```python
from build123d import *

# Parameters (mm, degrees)
BOSS_EXTRUDE1_DEPTH = 127
SKETCH4_W           = 31.75
SKETCH4_H           = 76.2
CUT_EXTRUDE3_DEPTH  = 63.5
SKETCH5_W           = 31.75
SKETCH5_H           = 76.2
CUT_EXTRUDE4_DEPTH  = 63.246
CUT_EXTRUDE6_DEPTH  = 69.85
CUT_EXTRUDE8_DEPTH  = 69.85
SKETCH9_R           = 4.7625
CUT_EXTRUDE9_DEPTH  = 461.057390442


with BuildPart() as part:
    # Sketch1 → Boss-Extrude1 (new body)
    with BuildSketch(Plane.XY):
        Polygon((63.5, -381), (63.5, 381), (31.75, 381), (31.75, 431.8), (-31.75, 431.8), (-31.75, 381), (-63.5, 381), (-63.5, -381), align=None)
    extrude(amount=-BOSS_EXTRUDE1_DEPTH)

    # Sketch4 → Cut-Extrude3 (cut)
    with BuildSketch(Plane.ZY.offset(63.5)):
        with Locations((-47.625, -215.9)):
            Rectangle(SKETCH4_W, SKETCH4_H)
    extrude(amount=-CUT_EXTRUDE3_DEPTH, mode=Mode.SUBTRACT)

    # Sketch5 → Cut-Extrude4 (cut)
    with BuildSketch(Plane(origin=(0, 0, -127), x_dir=(-1, 0, 0), z_dir=(0, 0, -1))):
        with Locations((-15.875, -215.9)):
            Rectangle(SKETCH5_W, SKETCH5_H)
    extrude(amount=-CUT_EXTRUDE4_DEPTH, mode=Mode.SUBTRACT)

    # Sketch7 → Cut-Extrude6 (cut)
    with BuildSketch(Plane(origin=(63.5, 0, 0), x_dir=(0, 0, -1), z_dir=(1, 0, 0))):
        with BuildLine():
            ThreePointArc((100.0125, -234.95), (98.617596045, -231.582403955), (95.25, -230.1875))
            Line((95.25, -230.1875), (95.25, -239.7125))
            ThreePointArc((95.25, -239.7125), (98.617596045, -238.317596045), (100.0125, -234.95))
        make_face()
        with BuildLine():
            Line((95.25, -239.7125), (95.25, -230.1875))
            ThreePointArc((95.25, -230.1875), (90.4875, -234.95), (95.25, -239.7125))
        make_face()
        with BuildLine():
            ThreePointArc((100.0125, -196.85), (98.617596045, -193.482403955), (95.25, -192.0875))
            Line((95.25, -192.0875), (95.25, -201.6125))
            ThreePointArc((95.25, -201.6125), (98.617596045, -200.217596045), (100.0125, -196.85))
        make_face()
        with BuildLine():
            Line((95.25, -201.6125), (95.25, -192.0875))
            ThreePointArc((95.25, -192.0875), (90.4875, -196.85), (95.25, -201.6125))
        make_face()
    extrude(amount=-CUT_EXTRUDE6_DEPTH, mode=Mode.SUBTRACT)

    # Sketch8 → Cut-Extrude8 (cut)
    with BuildSketch(Plane.XY):
        with BuildLine():
            ThreePointArc((-26.9875, -234.95), (-28.382403955, -231.582403955), (-31.75, -230.1875))
            Line((-31.75, -230.1875), (-31.75, -239.7125))
            ThreePointArc((-31.75, -239.7125), (-28.382403955, -238.317596045), (-26.9875, -234.95))
        make_face()
        with BuildLine():
            Line((-31.75, -239.7125), (-31.75, -230.1875))
            ThreePointArc((-31.75, -230.1875), (-36.5125, -234.95), (-31.75, -239.7125))
        make_face()
        with BuildLine():
            ThreePointArc((-26.9875, -196.85), (-28.382403955, -193.482403955), (-31.75, -192.0875))
            Line((-31.75, -192.0875), (-31.75, -201.6125))
            ThreePointArc((-31.75, -201.6125), (-28.382403955, -200.217596045), (-26.9875, -196.85))
        make_face()
        with BuildLine():
            Line((-31.75, -201.6125), (-31.75, -192.0875))
            ThreePointArc((-31.75, -192.0875), (-36.5125, -196.85), (-31.75, -201.6125))
        make_face()
    extrude(amount=-CUT_EXTRUDE8_DEPTH, mode=Mode.SUBTRACT)

    # Sketch9 → Cut-Extrude9 (cut, through all)
    with BuildSketch(Plane.ZY.offset(31.75)):
        with Locations(Location((-95.25, 406.4, 0), (0, 0, 270))):
            Circle(SKETCH9_R)
        with Locations(Location((-31.75, 406.4, 0), (0, 0, 270))):
            Circle(SKETCH9_R)
    extrude(amount=-CUT_EXTRUDE9_DEPTH, mode=Mode.SUBTRACT)


solid = part.part
```
For this review, take the finished solid that the model builds, in its own axes (mm). A direction names the side the tool comes from. Round coordinates to 2 decimals unless told otherwise and drop trailing zeros. Order: outer loops, then holes, each group sorted by start corner. A loop starts at its lowest first (then second) coordinate and runs counter-clockwise, first axis right, second up. Notation, with made-up numbers: (68.25, 71.25) -> (104.25, 71.25) arc R20 ccw to (104.25, 91.25) -> close; hole circle Ø2 at (-30, 13). An arc over 180 degrees is marked (long way). Use a Markdown table: item, result.
Item 1: Machinability: for faces 1 (the flat face through (16, -215, -63.754)), 2 (the flat face through (48, 381, -63)), 3 (the flat face through (-32, -177.8, -48)), which of the approach directions +Z, -Z, +X, -X, +Y, -Y give a long, thin tool a straight path to every point of the face, cutting with its end or side? Answer none if there is none.
Resolved:
| item | result |
|---|---|
| face 1 | -Z |
| face 2 | +Z, -Z, +X, +Y |
| face 3 | -X |
Item 2: Take a section at B-B (x = -15). State how many separate pieces and enclosed holes the cut face has, plus the area to 3 significant figures.
Resolved:
| item | result |
|---|---|
| separate pieces | 1 |
| enclosed holes | 3 |
| area | 101,000 mm² |
Item 3: For line 1 along Z through (x, y) = (-6, 406.4); line 2 along Y through (x, z) = (-54, -61); line 3 along Z through (x, y) = (-41, -237.5), list the stretches that pass through material, from the lowest coordinate up. Write a range as [from, to].
Resolved:
| item | result |
|---|---|
| line 1 | z = [-127, -100.01], [-90.49, -36.51], [-26.99, 0] |
| line 2 | y = [-381, -254], [-177.8, 381] |
| line 3 | z = [-127, -63.5], [-31.75, 0] |
Item 4: Take a section at A-A (z = -48). State the section outline as (x, y) points.
Resolved:
| item | result |
|---|---|
| outline | (-63.5, -381) -> (63.5, -381) -> (63.5, 381) -> (31.75, 381) -> (31.75, 431.8) -> (-31.75, 431.8) -> (-31.75, 381) -> (-63.5, 381) -> (-63.5, -177.8) -> (0, -177.8) -> (0, -254) -> (-63.5, -254) -> close |
Item 5: Draft analysis for pull direction X (two halves, no side actions). For faces 4 (the flat face through (31.75, 406, -63)), 5 (the flat face through (16, -254, -96)), 6 (the flat face through (31.75, -216, -96)), 7 (the flat face through (-1, -381, -63)), state which applies: +X half, -X half, draft (parallel to the pull), parting line (faces both ways), or undercut.
Resolved:
| item | result |
|---|---|
| face 4 | +X half |
| face 5 | undercut |
| face 6 | undercut |
| face 7 | draft |
Item 6: For pin 1 (12.5 mm diameter, centred on y = 406.4, z = -31.75, fed in from +X); pin 2 (12.5 mm diameter, centred on y = 406.4, z = -95.25, fed in from -X); pin 3 (2 mm diameter, centred on x = -39.5, z = -90, fed in from +Y), all flat-tipped, find the tip position at first contact; note any pin that passes through.
Resolved:
| item | result |
|---|---|
| pin 1 | stops at x = 31.75 |
| pin 2 | stops at x = -31.75 |
| pin 3 | stops at y = 381 |
Item 7: Take a section at D-D (x = -51). State the section outline as (y, z) points.
Resolved:
| item | result |
|---|---|
| outline | (-381, -127) -> (381, -127) -> (381, 0) -> (-381, 0) -> close; hole (-254, -63.5) -> (-177.8, -63.5) -> (-177.8, -31.75) -> (-254, -31.75) -> close |
